```python
from build123d import *

# Parameters (mm, degrees)
SKETCH1_W                      = 100
SKETCH1_H                      = 100
BASE_FLANGE1_DEPTH             = 1.5
EDGE_FLANGE1_STRIP_W           = 10
EDGE_FLANGE1_STRIP_H           = 1.5
EDGE_FLANGE1_STRIP_CUT_DEPTH   = 100
EDGE_FLANGE1_STRIP_2_W         = 10
EDGE_FLANGE1_STRIP_2_H         = 1.5
EDGE_FLANGE1_STRIP_CUT_2_DEPTH = 100
EDGE_FLANGE1_DEPTH             = 100
EDGE_FLANGE1_BEND_DEPTH        = 100
EDGE_FLANGE2_STRIP_W           = 10
EDGE_FLANGE2_STRIP_H           = 1.5
EDGE_FLANGE2_STRIP_CUT_DEPTH   = 100
EDGE_FLANGE2_STRIP_2_W         = 10
EDGE_FLANGE2_STRIP_2_H         = 1.5
EDGE_FLANGE2_STRIP_CUT_2_DEPTH = 100
EDGE_FLANGE2_DEPTH             = 100
EDGE_FLANGE2_BEND_DEPTH        = 100
F_6_0_6_DIAMETER_HOLE1_D       = 6
CHAMFER1_SIZE                  = 6
SKETCH20_R                     = 6
BOSS_EXTRUDE1_DEPTH            = 1.5
SKETCHED_START                 = 57.64041
SKETCHED_BEND1_OUTLINE_W       = 24
SKETCHED_BEND1_OUTLINE_H       = 1.5
SKETCHED_BEND1_DEPTH           = 35.35959
SKETCHED_START_2               = 54.5
SKETCHED_BEND1_2_OUTLINE_R     = 6
SKETCHED_BEND1_2_DEPTH         = 3.5
SKETCHED_START_3               = -12
SKETCHED_BEND1_3_DEPTH         = 24


with BuildPart() as part:
    # Base-Flange1: sheet metal written as solids
    # Sketch1 → Base-Flange1 (new body)
    with BuildSketch(Plane(origin=(0, 0, 0), x_dir=(1, 0, 0), z_dir=(0, 1, 0))):
        Rectangle(SKETCH1_W, SKETCH1_H)
    extrude(amount=-BASE_FLANGE1_DEPTH)

    # Edge-Flange1: sheet metal written as solids
    # Edge-Flange1 strip (on a plane across the edge) → Edge-Flange1 strip cut (cut)
    with BuildSketch(Plane(origin=(-50, 0, -50), x_dir=(1, 0, 0), z_dir=(0, 0, 1))):
        with Locations((-1.5, -0.75)):
            Rectangle(EDGE_FLANGE1_STRIP_W, EDGE_FLANGE1_STRIP_H)
    extrude(amount=EDGE_FLANGE1_STRIP_CUT_DEPTH, mode=Mode.SUBTRACT)

    # Edge-Flange1 strip 2 (on a plane across the edge) → Edge-Flange1 strip cut 2 (cut)
    with BuildSketch(Plane(origin=(50, 0, 50), x_dir=(-1, 0, 0), z_dir=(0, 0, -1))):
        with Locations((-1.5, -0.75)):
            Rectangle(EDGE_FLANGE1_STRIP_2_W, EDGE_FLANGE1_STRIP_2_H)
    extrude(amount=EDGE_FLANGE1_STRIP_CUT_2_DEPTH, mode=Mode.SUBTRACT)

    # Edge-Flange1 section (on a plane across the edge) → Edge-Flange1 (add)
    with BuildSketch(Plane(origin=(-50, 0, -50), x_dir=(1, 0, 0), z_dir=(0, 0, 1))):
        with BuildLine():
            Line((0, 2), (0, 33.5))
            Line((0, 33.5), (1.5, 33.5))
            Line((1.5, 33.5), (1.5, 2))
            ThreePointArc((1.5, 2), (2.085786438, 0.585786438), (3.5, 0))
            Line((3.5, 0), (3.5, -1.5))
            ThreePointArc((3.5, -1.5), (1.025126266, -0.474873734), (0, 2))
        make_face()
    extrude(amount=EDGE_FLANGE1_DEPTH)

    # Edge-Flange1 section 2 (on a plane across the edge) → Edge-Flange1 bend (add)
    with BuildSketch(Plane(origin=(50, 0, 50), x_dir=(-1, 0, 0), z_dir=(0, 0, -1))):
        with BuildLine():
            Line((0, 2), (0, 33.5))
            Line((0, 33.5), (1.5, 33.5))
            Line((1.5, 33.5), (1.5, 2))
            ThreePointArc((1.5, 2), (2.085786438, 0.585786438), (3.5, 0))
            Line((3.5, 0), (3.5, -1.5))
            ThreePointArc((3.5, -1.5), (1.025126266, -0.474873734), (0, 2))
        make_face()
    extrude(amount=EDGE_FLANGE1_BEND_DEPTH)

    # Edge-Flange2: sheet metal written as solids
    # Edge-Flange2 strip (on a plane across the edge) → Edge-Flange2 strip cut (cut)
    with BuildSketch(Plane(origin=(-50, 33.5, 50), x_dir=(0, -1, 0), z_dir=(0, 0, -1))):
        with Locations((-1.5, -0.75)):
            Rectangle(EDGE_FLANGE2_STRIP_W, EDGE_FLANGE2_STRIP_H)
    extrude(amount=EDGE_FLANGE2_STRIP_CUT_DEPTH, mode=Mode.SUBTRACT)

    # Edge-Flange2 strip 2 (on a plane across the edge) → Edge-Flange2 strip cut 2 (cut)
    with BuildSketch(Plane(origin=(50, 33.5, -50), x_dir=(0, -1, 0), z_dir=(0, 0, 1))):
        with Locations((-1.5, -0.75)):
            Rectangle(EDGE_FLANGE2_STRIP_2_W, EDGE_FLANGE2_STRIP_2_H)
    extrude(amount=EDGE_FLANGE2_STRIP_CUT_2_DEPTH, mode=Mode.SUBTRACT)

    # Edge-Flange2 section (on a plane across the edge) → Edge-Flange2 (add)
    with BuildSketch(Plane(origin=(-50, 33.5, 50), x_dir=(0, -1, 0), z_dir=(0, 0, -1))):
        with BuildLine():
            Line((0, 2), (0, 23.5))
            Line((0, 23.5), (1.5, 23.5))
            Line((1.5, 23.5), (1.5, 2))
            ThreePointArc((1.5, 2), (2.085786438, 0.585786438), (3.5, 0))
            Line((3.5, 0), (3.5, -1.5))
            ThreePointArc((3.5, -1.5), (1.025126266, -0.474873734), (0, 2))
        make_face()
    extrude(amount=EDGE_FLANGE2_DEPTH)

    # Edge-Flange2 section 2 (on a plane across the edge) → Edge-Flange2 bend (add)
    with BuildSketch(Plane(origin=(50, 33.5, -50), x_dir=(0, -1, 0), z_dir=(0, 0, 1))):
        with BuildLine():
            Line((0, 2), (0, 23.5))
            Line((0, 23.5), (1.5, 23.5))
            Line((1.5, 23.5), (1.5, 2))
            ThreePointArc((1.5, 2), (2.085786438, 0.585786438), (3.5, 0))
            Line((3.5, 0), (3.5, -1.5))
            ThreePointArc((3.5, -1.5), (1.025126266, -0.474873734), (0, 2))
        make_face()
    extrude(amount=EDGE_FLANGE2_BEND_DEPTH)

    # Ø6.0 (6) Diameter Hole1 (through all)
    with Locations(Plane(origin=(0, 33.5, 0), x_dir=(1, 0, 0), z_dir=(0, 1, 0))):
        with Locations((-63.5, 35), (-63.5, -35), (63.5, 35), (63.5, -35)):
            Hole(F_6_0_6_DIAMETER_HOLE1_D / 2)

    # Chamfer1
    chamfer1_edges = [part.edges().sort_by_distance(p)[0] for p in [
        (-73.5, 32.75, 50),
        (-73.5, 32.75, -50),
        (73.5, 32.75, -50),
        (73.5, 32.75, 50),
    ]]
    chamfer(chamfer1_edges, length=CHAMFER1_SIZE)

    # Sketch20 → Boss-Extrude1 (add)
    # profile 1 of 2: a face of its own
    with BuildSketch(Plane(origin=(0, 0, 0), x_dir=(1, 0, 0), z_dir=(0, 1, 0))):
        with BuildLine():
            Line((-12, 50), (-12, 80))
            ThreePointArc((-12, 80), (0, 92), (12, 80))
            Line((12, 80), (12, 50))
            Line((12, 50), (-12, 50))
        make_face()
        with Locations(Location((0, 80, 0), (0, 0, 270))):
            Circle(SKETCH20_R, mode=Mode.SUBTRACT)
    # profile 2 of 2: a face of its own
    with BuildSketch(Plane(origin=(0, 0, 0), x_dir=(1, 0, 0), z_dir=(0, 1, 0))):
        with BuildLine():
            Line((12, -50), (-12, -50))
            Line((-12, -50), (-12, -80))
            ThreePointArc((-12, -80), (0, -92), (12, -80))
            Line((12, -80), (12, -50))
        make_face()
        with Locations(Location((0, -80, 0), (0, 0, 90))):
            Circle(SKETCH20_R, mode=Mode.SUBTRACT)
    extrude(amount=-BOSS_EXTRUDE1_DEPTH)

    # Sketched Bend1: read off the stored shape, not the designer's step
    # Sketched Bend1 outline → Sketched Bend1 (cut)
    with BuildSketch(Plane.XY.offset(SKETCHED_START)):
        with Locations((0, -0.75)):
            Rectangle(SKETCHED_BEND1_OUTLINE_W, SKETCHED_BEND1_OUTLINE_H)
    extrude(amount=SKETCHED_BEND1_DEPTH, mode=Mode.SUBTRACT)

    # Sketched Bend1 2 outline → Sketched Bend1 2 (add)
    with BuildSketch(Plane.XY.offset(SKETCHED_START_2)):
        with BuildLine():
            Line((-12, -1.5), (-12, -24.680310101))
            ThreePointArc((-12, -24.680310101), (0, -36.680310101), (12, -24.680310101))
            Line((12, -24.680310101), (12, -1.5))
            Line((12, -1.5), (-12, -1.5))
        make_face()
        with Locations((0, -24.680310101)):
            Circle(SKETCHED_BEND1_2_OUTLINE_R, mode=Mode.SUBTRACT)
    extrude(amount=SKETCHED_BEND1_2_DEPTH)

    # Sketched Bend1 3 outline → Sketched Bend1 3 (cut)
    with BuildSketch(Plane.YZ.offset(SKETCHED_START_3)):
        with BuildLine():
            ThreePointArc((-1.5, 54.5), (-2.085786438, 55.914213562), (-3.5, 56.5))
            Line((-3.5, 56.5), (-38, 56.5))
            Line((-38, 56.5), (-38, 54.5))
            Line((-38, 54.5), (-1.5, 54.5))
        make_face()
        with BuildLine():
            Line((-38, 59), (-38, 58.000000005))
            Line((-38, 58.000000005), (-3.5, 58))
            ThreePointArc((-3.5, 58), (-1.025126266, 56.974873734), (0, 54.5))
            Line((0, 54.5), (0, 53))
            Line((0, 53), (1, 53))
            Line((1, 53), (1, 57.64041))
            Line((1, 57.64041), (-1.5, 57.64041))
            Line((-1.5, 57.64041), (-1.5, 59))
            Line((-1.5, 59), (-38, 59))
        make_face()
    extrude(amount=SKETCHED_BEND1_3_DEPTH, mode=Mode.SUBTRACT)


solid = part.part
```
Can you work these out from the model? Positions are in its coordinate system, mm. A direction names the side the tool comes from. Round coordinates to 2 decimals unless told otherwise and drop trailing zeros. Loops run counter-clockwise (first coordinate to the right, second up) from the corner with the lowest first, then second, coordinate; pieces in that order, holes last.
Item 1: Suppose I cut it at B-B, the plane z = -35. Write out the boundary of the cut face in (x, y).
Item 2: Will these pins go through, and if not, where does the flat tip stop? pin 1 Ø4 at (y, z) = (-4.5, -23) entering from -X; pin 2 Ø22.5 at (y, z) = (14.5, 14.5) entering from +X; pin 3 Ø22.5 at (y, z) = (16.5, -16.5) entering from -X; pin 4 Ø12 at (x, z) = (20, -25) entering from -Y.
Item 3: Suppose I cut it at C-C, the plane y = 6. Write out the boundary of the cut face in (x, z), then the cut area to 3 significant figures.
Item 4: Please list where these lines run through material, in increasing order: L1, parallel to Z at x = -63.5, y = 32.7; L2, parallel to X at y = 14, z = -29; L3, parallel to X at y = 33.15, z = -35.
Item 5: If we mould it in two halves opening along X, with no side actions, what happens to faces 1 (the flat face through (-63, 32, 1)), 2 (the flat face through (-70.5, 32.8, 47)), 3 (the flat face through (48.5, 16, 1))? For each: +X half, -X half, draft (parallel to the pull), parting line (faces both ways), or undercut.
Item 6: Suppose I cut it at D-D, the plane z = -7. Write out the boundary of the cut face in (x, y), then the cut area to 3 significant figures.
Item 7: Suppose I cut it at A-A, the plane x = 63.5. Write out the boundary of the cut face in (y, z), then the cut area to 3 significant figures.
Item 8: Which directions (+Z, -Z, +X, -X, +Y, -Y) give clear straight access to the entire face, cutting with the end or side of a thin tool? Please do faces 4 (the flat face through (12, -10, 57)), 5 (the flat face through (50, 16, 1)), 6 (the flat face through (-1, -1.5, -3)).
Reported:
1. outline: (-73.5, 32) - (-66.5, 32) - (-66.5, 33.5) - (-73.5, 33.5) - close; (-60.5, 32) - (-52, 32) arc R2 cw to (-50, 30) - (-50, 2) arc R3.5 ccw to (-46.5, -1.5) - (46.5, -1.5) arc R3.5 ccw to (50, 2) - (50, 30) arc R2 cw to (52, 32) - (60.5, 32) - (60.5, 33.5) - (52, 33.5) arc R3.5 ccw to (48.5, 30) - (48.5, 2) arc R2 cw to (46.5, 0) - (-46.5, 0) arc R2 cw to (-48.5, 2) - (-48.5, 30) arc R3.5 ccw to (-52, 33.5) - (-60.5, 33.5) - close; (66.5, 32) - (73.5, 32) - (73.5, 33.5) - (66.5, 33.5) - close
2. pin 1: passes through
2. pin 2: stops at x = 50
2. pin 3: stops at x = -50
2. pin 4: stops at y = -1.5
3. outline: (-50, -50) - (-48.5, -50) - (-48.5, 50) - (-50, 50) - close; (48.5, -50) - (50, -50) - (50, 50) - (48.5, 50) - close
3. area: 300 mm2
4. L1: z = -50 to -38, -32 to 32, 38 to 50
4. L2: x = -50 to -48.5, 48.5 to 50
4. L3: x = -73.5 to -66.5, -60.5 to -50.47, 50.47 to 60.5, 66.5 to 73.5
5. face 1: draft
5. face 2: -X half
5. face 3: undercut
6. outline: (-73.5, 32) - (-52, 32) arc R2 cw to (-50, 30) - (-50, 2) arc R3.5 ccw to (-46.5, -1.5) - (46.5, -1.5) arc R3.5 ccw to (50, 2) - (50, 30) arc R2 cw to (52, 32) - (73.5, 32) - (73.5, 33.5) - (52, 33.5) arc R3.5 ccw to (48.5, 30) - (48.5, 2) arc R2 cw to (46.5, 0) - (-46.5, 0) arc R2 cw to (-48.5, 2) - (-48.5, 30) arc R3.5 ccw to (-52, 33.5) - (-73.5, 33.5) - close
6. area: 314 mm2
7. outline: (32, -50) - (33.5, -50) - (33.5, -38) - (32, -38) - close; (32, -32) - (33.5, -32) - (33.5, 32) - (32, 32) - close; (32, 38) - (33.5, 38) - (33.5, 50) - (32, 50) - close
7. area: 132 mm2
8. face 4: +Z, +X, +Y, -Y
8. face 5: +Z, -Z, +X, -Y
8. face 6: -Z, +X, -X, -Y
